Check sheet for the drawn part. Datum: minimum x, y, z corner. Units: mm. Give positions to 0.01 mm unless a question says otherwise; leave off trailing zeros. Write each loop counter-clockwise with the first axis right and the second up, starting at its lowest first coordinate (ties: lowest second). Pieces come first, ordered by that corner, then holes.
(1) Cross-section at B-B (z = 2.5). Record the boundary of the cut face in (x, y), and give its area (3 significant figures).
(2) Cross-section at C-C (y = 4.75). Record the boundary of the cut face in (x, z), and give its area (3 significant figures).
(3) Mould release check, pull along Z, two halves, no side actions. Record for the marked faces 1, 2 and 3: +Z half, -Z half, draft (parallel to the pull), parting line (faces both ways), or undercut.
(4) Depth check by flat-ended pin: P1, Ø0.5, axis at x = 10.5, z = 0.5, coming from the +Y side; P2, Ø3, axis at x = 16, y = 4, coming from the -Z side; P3, Ø5, axis at x = 11, y = 5, coming from the +Z side; P4, Ø2.5, axis at y = 9, z = 1.5, coming from the +X side. Enter the tip coordinate at first touch or a pass-through.
(5) Thickness scan on line 1 along Y through (x, z) = (17.35, 2.5); line 2 along X through (y, z) = (11.5, 2.8); line 3 along Z through (x, y) = (18.95, 9.5). Record the ranges inside material, lowest first.
(6) Cross-section at A-A (z = 4.5). Record the boundary of the cut face in (x, y), and give its area (3 significant figures).
(7) Cross-section at D-D (x = 15.5). Record the boundary of the cut face in (y, z) (3 decimals).
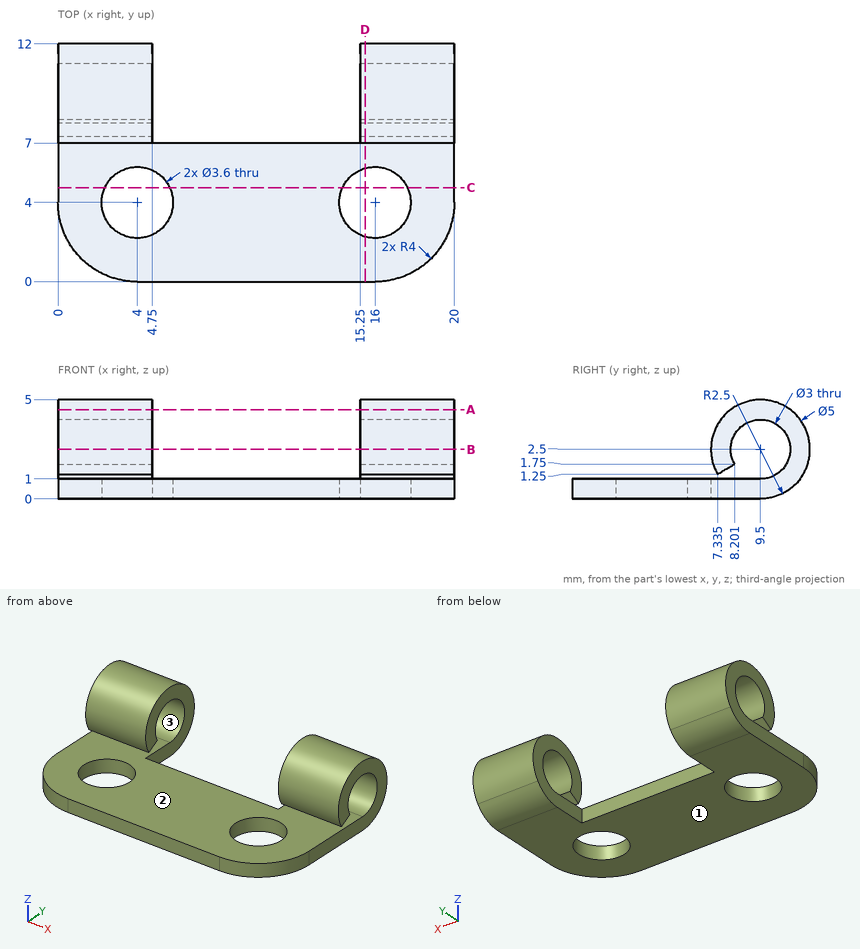
Reply:
1. outline: (0, 7) - (4.75, 7) - (4.75, 8) - (0, 8) - close; (0, 11) - (4.75, 11) - (4.75, 12) - (0, 12) - close; (15.25, 7) - (20, 7) - (20, 8) - (15.25, 8) - close; (15.25, 11) - (20, 11) - (20, 12) - (15.25, 12) - close
1. area: 19.0 mm2
2. outline: (0, 0) - (2.36, 0) - (2.36, 1) - (0, 1) - close; (5.64, 0) - (14.36, 0) - (14.36, 1) - (5.64, 1) - close; (17.64, 0) - (20, 0) - (20, 1) - (17.64, 1) - close
2. area: 13.5 mm2
3. face 1: -Z half
3. face 2: undercut
3. face 3: undercut
4. P1: stops at y = 7
4. P2: passes through
4. P3: stops at z = 1
4. P4: stops at x = 20
5. line 1: y = 7 to 8, 11 to 12
5. line 2: x = 0 to 4.75, 15.25 to 20
5. line 3: z = 0 to 1, 4 to 5
6. outline: (0, 8) - (4.75, 8) - (4.75, 11) - (0, 11) - close; (15.25, 8) - (20, 8) - (20, 11) - (15.25, 11) - close
6. area: 28.5 mm2
7. outline: (0, 0) - (2.271, 0) - (2.271, 1) - (0, 1) - close; (5.729, 0) - (9.5, 0) arc R2.5 ccw (long way) to (7.335, 1.25) - (8.201, 1.75) arc R1.5 cw (long way) to (9.5, 1) - (5.729, 1) - close
